from build123d import *

# Parameters (mm, degrees)
F0_W     = 25
F0_H     = 25
F1_DEPTH = 12.5
F2_SIZE  = 3.5


with BuildPart() as f1:
    # F0 (on Top) → F1 (new body, symmetric)
    with BuildSketch(Plane.XY):
        Rectangle(F0_W, F0_H)
    extrude(amount=F1_DEPTH, both=True)

    # F2
    f2_edges = [f1.edges().sort_by_distance(p)[0] for p in [
        (0, -12.5, -12.5),
        (12.5, -12.5, 0),
        (0, -12.5, 12.5),
        (-12.5, -12.5, 0),
        (12.5, 0, 12.5),
        (0, 12.5, 12.5),
        (-12.5, 0, 12.5),
        (-12.5, 12.5, 0),
        (-12.5, 0, -12.5),
        (12.5, 0, -12.5),
        (12.5, 12.5, 0),
        (0, 12.5, -12.5),
    ]]
    chamfer(f2_edges, length=F2_SIZE)


solid = f1.part
Here's how the part is built. I have some questions about the finished solid (model axes, mm). Give positions to 0.01 mm unless a question says otherwise; leave off trailing zeros. Loops run counter-clockwise (first coordinate to the right, second up) from the corner with the lowest first, then second, coordinate; pieces in that order, holes last. Notation, with made-up numbers: (89.25, 73.25) -> (103.25, 73.25) arc R12 ccw to (103.25, 95.25) -> close; hole circle Ø2 at (25, 64.5). An arc over 180 degrees is marked (long way). Answer as a JSON object with one key per item and string values. Group by question number.
Item 1: Imagine slicing it at A-A on x = -8.5. Write out the boundary of the cut face in (y, z).
Item 2: I need wall thicknesses on L1, parallel to X at y = -10, z = 1.5; L2, parallel to Z at x = -9.5, y = -7.5; L3, parallel to X at y = -6.75, z = 9.25. Which ranges of each line are inside material? Lowest first, please.
Answer list:
{
 "1": {"outline": "(-12.5, -9) -> (-9, -12.5) -> (9, -12.5) -> (12.5, -9) -> (12.5, 9) -> (9, 12.5) -> (-9, 12.5) -> (-12.5, 9) -> close"},
 "2": {"L1": "x = -11.5 to 11.5", "L2": "z = -12 to 12", "L3": "x = -12.25 to 12.25"}
}
